```python
from build123d import *

# Parameters (mm, degrees)
SKETCH2_W           = 110
SKETCH2_H           = 90
BOSS_EXTRUDE2_DEPTH = 60
SKETCH5_W           = 92
SKETCH5_H           = 72
CUT_EXTRUDE3_DEPTH  = 3
SKETCH6_W           = 92
SKETCH6_H           = 72
CUT_EXTRUDE4_DEPTH  = 10
SKETCH7_W           = 82
SKETCH7_H           = 62
CUT_EXTRUDE5_DEPTH  = 60


with BuildPart() as part:
    # Sketch2 → Boss-Extrude2 (new body)
    with BuildSketch(Plane(origin=(0, 0, 0), x_dir=(1, 0, 0), z_dir=(0, 1, 0))):
        with Locations((55, 45)):
            Rectangle(SKETCH2_W, SKETCH2_H)
    extrude(amount=BOSS_EXTRUDE2_DEPTH)

    # Sketch5 → Cut-Extrude3 (cut)
    with BuildSketch(Plane(origin=(0, 60, 0), x_dir=(1, 0, 0), z_dir=(0, 1, 0))):
        with Locations((55, 45)):
            Rectangle(SKETCH5_W, SKETCH5_H)
    extrude(amount=-CUT_EXTRUDE3_DEPTH, mode=Mode.SUBTRACT)

    # Sketch6 → Cut-Extrude4 (cut)
    with BuildSketch(Plane.XZ):
        with Locations((55, -45)):
            Rectangle(SKETCH6_W, SKETCH6_H)
    extrude(amount=-CUT_EXTRUDE4_DEPTH, mode=Mode.SUBTRACT)

    # Sketch7 → Cut-Extrude5 (cut)
    with BuildSketch(Plane(origin=(0, 57, 0), x_dir=(1, 0, 0), z_dir=(0, 1, 0))):
        with Locations((55, 45)):
            Rectangle(SKETCH7_W, SKETCH7_H)
    extrude(amount=-CUT_EXTRUDE5_DEPTH, mode=Mode.SUBTRACT)


solid = part.part
```
Design review of the part built by this model. Coordinates are the model's own, in mm. A direction names the side the tool comes from. Round coordinates to 2 decimals unless told otherwise and drop trailing zeros. Write each loop counter-clockwise with the first axis right and the second up, starting at its lowest first coordinate (ties: lowest second). Pieces come first, ordered by that corner, then holes. Notation, with made-up numbers: (14, 14.5) -> (54, 14.5) arc R22 cw to (54, 53.5) -> close; hole circle Ø3 at (75.5, 74). An arc over 180 degrees is marked (long way). Answer in a Markdown table with one row per item.
Q1. Draft analysis for pull direction Z (two halves, no side actions). For faces 6 (the face through (101, 5, -46)), 7 (the face through (54, 30, 0)), 8 (the face through (54, 0, -86)), 9 (the face through (54, 30, -90)), state which applies: +Z half, -Z half, draft (parallel to the pull), parting line (faces both ways), or undercut.
The answers:
| item | result |
|---|---|
| face 6 | undercut |
| face 7 | +Z half |
| face 8 | draft |
| face 9 | -Z half |
Q2. Take a section at A-A, the plane z = -52. State the section outline as (x, y) points.
The answers:
| item | result |
|---|---|
| outline | (0, 0) -> (9, 0) -> (9, 10) -> (14, 10) -> (14, 57) -> (9, 57) -> (9, 60) -> (0, 60) -> close; (96, 10) -> (101, 10) -> (101, 0) -> (110, 0) -> (110, 60) -> (101, 60) -> (101, 57) -> (96, 57) -> close |
Q3. To check wall thickness, follow L1, parallel to X at y = 56, z = -60; L2, parallel to Z at x = 53, y = 28.5; L3, parallel to X at y = 5.5, z = -24. State the ranges of each line that lie inside material, in increasing order. Write a range as [from, to].
The answers:
| item | result |
|---|---|
| L1 | [0, 14], [96, 110] |
| L2 | [-90, -76], [-14, 0] |
| L3 | [0, 9], [101, 110] |
Q4. Take a section at D-D, the plane x = 12. State the section outline as (y, z) points, then the cut area to 3 significant figures.
The answers:
| item | result |
|---|---|
| outline | (0, -90) -> (60, -90) -> (60, -81) -> (57, -81) -> (57, -9) -> (60, -9) -> (60, 0) -> (0, 0) -> (0, -9) -> (10, -9) -> (10, -81) -> (0, -81) -> close |
| area | 4,460 mm² |
Q5. Take a section at B-B, the plane y = 18. State the section outline as (x, z) points.
The answers:
| item | result |
|---|---|
| outline | (0, -90) -> (110, -90) -> (110, 0) -> (0, 0) -> close; hole (14, -76) -> (96, -76) -> (96, -14) -> (14, -14) -> close |
Q6. For faces 1 (the face through (54, 34, -14)), 2 (the face through (45, 10, -77)), 3 (the face through (0, 30, -44)), 4 (the face through (54, 59, -9)), 5 (the face through (54, 60, -86)), list the 3-axis set-ups (+Z, -Z, +X, -X, +Y, -Y) from which the entire face can be reached by the end or side of a thin tool; tool diameter is ignored.
The answers:
| item | result |
|---|---|
| face 1 | +Y, -Y |
| face 2 | -Y |
| face 3 | +Z, -Z, -X, +Y, -Y |
| face 4 | +Y |
| face 5 | +Z, -Z, +X, -X, +Y |
Q7. Clearance check with flat-ended pins moving along their axes: pin 1 Ø10 at (x, y) = (85, 21.5) entering from +Z; pin 2 Ø6 at (x, z) = (34.5, -15.5) entering from -Y. State where each tip first meets the part, or that it passes through.
The answers:
| item | result |
|---|---|
| pin 1 | z = 0 |
| pin 2 | y = 10 |
Q8. Take a section at C-C, the plane x = 43. State the section outline as (y, z) points.
The answers:
| item | result |
|---|---|
| outline | (0, -90) -> (60, -90) -> (60, -81) -> (57, -81) -> (57, -76) -> (10, -76) -> (10, -81) -> (0, -81) -> close; (0, -9) -> (10, -9) -> (10, -14) -> (57, -14) -> (57, -9) -> (60, -9) -> (60, 0) -> (0, 0) -> close |
